The figure shows three views and two pictorial views of one solid part (mm, origin at its lowest corner). Answer the questions. Round coordinates to 2 decimals unless told otherwise and drop trailing zeros. Order: outer loops, then holes, each group sorted by start corner. A loop starts at its lowest first (then second) coordinate and runs counter-clockwise, first axis right, second up. Notation, with made-up numbers: (54, -36.5) - (71, -36.5) arc R38 ccw to (71, 1.5) - close; hole circle Ø9 at (9.25, -24). An arc over 180 degrees is marked (long way). One line per question, with ' | ' between items. Start each with the question number.
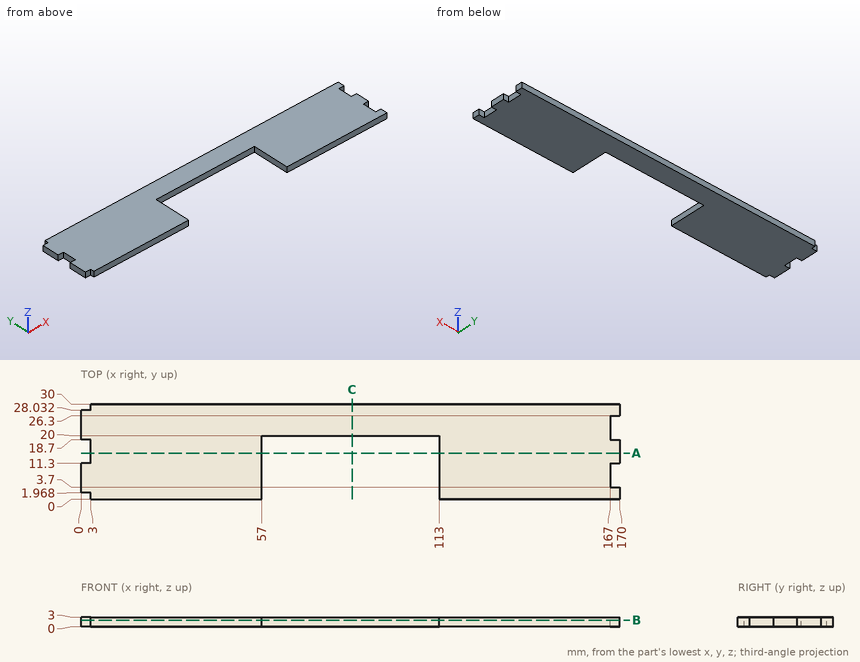
1) Straight lines are drawn through the part: line 1 (X direction, y = 1, z = 0.4); line 2 (X direction, y = 3.25, z = 0.4); line 3 (Y direction, x = 90, z = 2.1). For each, find the intervals that lie inside material, in ascending order.
2) Section C-C on x = 85.5 is taken. Give the vertices of the cut face in (y, z), and give its area (3 significant figures).
3) Section B-B on z = 2.05 is taken. Give the vertices of the cut face in (x, y).
4) Flat-ended cylindrical pins translate along their axes: pin 1 (0.9 mm diameter, centred on x = 1.5, z = 1, fed in from -Y); pin 2 (0.9 mm diameter, centred on y = 7, z = 1.5, fed in from +X); pin 3 (0.9 mm diameter, centred on x = 1, z = 2, fed in from +Y). Find the tip coordinate at first contact, or state that the pin passes through.
5) Section A-A on y = 14.5 is taken. Give the vertices of the cut face in (x, z).
Recorded:
1) line 1: x = 3 to 57, 113 to 170 | line 2: x = 0 to 57, 113 to 170 | line 3: y = 20 to 30
2) outline: (20, 0) - (30, 0) - (30, 3) - (20, 3) - close | area: 30.0 mm²
3) outline: (0, 1.97) - (3, 1.97) - (3, 0) - (57, 0) - (57, 20) - (113, 20) - (113, 0) - (170, 0) - (170, 3.7) - (167, 3.7) - (167, 11.3) - (170, 11.3) - (170, 18.7) - (167, 18.7) - (167, 26.3) - (170, 26.3) - (170, 30) - (3, 30) - (3, 28.03) - (0, 28.03) - (0, 18.7) - (3, 18.7) - (3, 11.3) - (0, 11.3) - close
4) pin 1: stops at y = 1.97 | pin 2: stops at x = 167 | pin 3: stops at y = 28.03
5) outline: (3, 0) - (57, 0) - (57, 3) - (3, 3) - close; (113, 0) - (170, 0) - (170, 3) - (113, 3) - close
